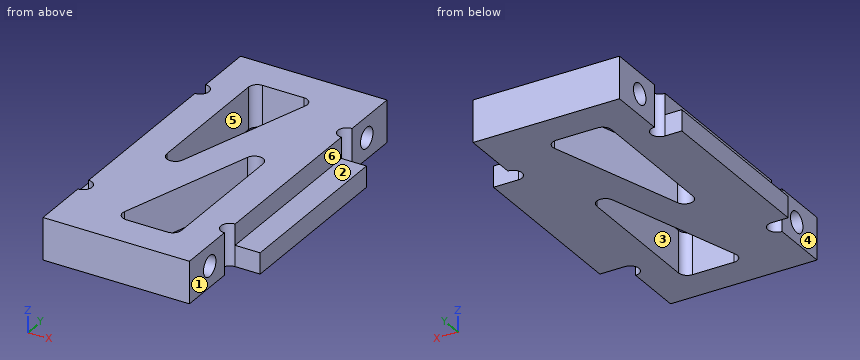
Autodesk Inventor part; units mm, degrees
ref_plane "YZ Plane" through (0, 0, 0) normal (1, 0, 0) x (0, 1, 0)
ref_plane "XZ Plane" through (0, 0, 0) normal (0, 1, 0) x (-1, 0, 0)
ref_plane "XY Plane" through (0, 0, 0) normal (0, 0, 1) x (1, 0, 0)
sketch "スケッチ1" plane through (0, 0, 0) normal (0, 0, 1) x (1, 0, 0)
  line L0 (-8.75, -19.5) -> (8.75, -19.5) construction
  line L1 (8.75, -19.5) -> (8.75, 19.5) construction
  line L2 (8.75, 19.5) -> (-8.75, 19.5) construction
  line L3 (-8.75, 19.5) -> (-8.75, -19.5) construction
  line L4 (-8.75, -19.5) -> (8.75, 19.5) construction
  line L5 (8.75, -19.5) -> (-8.75, 19.5) construction
  line L6 (-8.75, 10.5) -> (-8.75, 19.5) construction
  line L7 (-8.75, 19.5) -> (8.75, 19.5)
  line L8 (8.75, 19.5) -> (8.75, 10.5) construction
  line L9 (-8.75, 10.5) -> (-10.75, 10.5)
  line L10 (-10.75, 10.5) -> (-10.75, -10.5)
  line L11 (-10.75, -10.5) -> (-8.75, -10.5)
  line L12 (-8.75, -10.5) -> (-8.75, -19.5) construction
  line L13 (-8.75, -19.5) -> (8.75, -19.5)
  line L14 (8.75, -19.5) -> (8.75, -10.5) construction
  line L15 (8.75, -10.5) -> (11.75, -10.5)
  line L16 (11.75, -10.5) -> (11.75, 10.5)
  line L17 (11.75, 10.5) -> (8.75, 10.5)
  line L18 (0, 0) -> (11.75, 0) construction
  circle A0 centre (-8.75, 11.55) radius 1.05 construction
  circle A1 centre (-8.75, -11.55) radius 1.05 construction
  circle A2 centre (8.75, 11.55) radius 1.05 construction
  circle A3 centre (8.75, -11.55) radius 1.05 construction
  line L19 (-8.75, 19.5) -> (-8.75, 12.6)
  arc A4 (-8.75, 10.5) -> (-8.75, 12.6) centre (-8.75, 11.55) ccw
  arc A5 (-8.75, -12.6) -> (-8.75, -10.5) centre (-8.75, -11.55) ccw
  line L20 (-8.75, -12.6) -> (-8.75, -19.5)
  line L21 (8.75, 12.6) -> (8.75, 19.5)
  arc A6 (8.75, 12.6) -> (8.75, 10.5) centre (8.75, 11.55) ccw
  line L22 (8.75, -12.6) -> (8.75, -19.5)
  arc A7 (8.75, -10.5) -> (8.75, -12.6) centre (8.75, -11.55) ccw
  dimension "d21" = 2
  dimension "d23" = 3
  dimension "d30" = 17.5
  dimension "d48" = 9
  dimension "d49" = 39
  dimension "d50" = 2.1
extrude "押し出し1" add sketch "スケッチ1" along normal blind 5
sketch "スケッチ2" plane through (8.75, -19.5, 0) normal (1, 0, 0) x (0, 0, -1)
  line L0 (0, 0) -> (-5, 0)
  line L1 (0, 39) -> (-5, 39)
  point P0 (0, 19.5)
  point P1 (-2.5, 4)
  point P2 (-2.5, 35)
  point P3 (-2.5, 0)
  dimension "d53" = 4
  dimension "d54" = 4
hole "穴1" at (8.75, -15.5, 2.5) at (8.75, 15.5, 2.5) direction (-1, 0, 0) diameter 2.459 depth 2.5 tip angle 118
mirror "ミラー1" about plane through (0, 0, 0) normal (1, 0, 0) of "穴1"
sketch "スケッチ3" plane through (0, 0, 5) normal (0, 0, 1) x (1, 0, 0)
  line L0 (8.75, 12.6) -> (8.75, 19.5)
  line L1 (-8.75, 19.5) -> (-8.75, 12.6)
  line L2 (-13.3307, 15.6684) -> (-8.75, 15.6684)
  line L3 (-8.75, 15.6684) -> (-8.75, -16.7148)
  line L4 (-8.75, -16.7148) -> (-13.3307, -16.7148)
  line L5 (-13.3307, -16.7148) -> (-13.3307, 15.6684)
  line L6 (14.2214, 11.55) -> (8.75, 11.55)
  line L7 (8.75, 11.55) -> (8.75, -15.9078)
  line L8 (8.75, -15.9078) -> (14.2214, -15.9078)
  line L9 (14.2214, -15.9078) -> (14.2214, 11.55)
  point P0 (0, 0)
extrude "押し出し2" cut sketch "スケッチ3" against normal blind 2.5
sketch "スケッチ4" plane through (0, 0, 5) normal (0, 0, 1) x (1, 0, 0)
  line L0 (8.75, 12.6) -> (8.75, 19.5)
  line L1 (8.75, 19.5) -> (-8.75, 19.5)
  line L2 (-8.75, -12.6) -> (-8.75, -19.5)
  line L3 (-8.75, -19.5) -> (8.75, -19.5)
  line L4 (-4.75, 15.5) -> (4.75, 15.5) construction
  line L5 (4.75, 15.5) -> (4.75, -15.5) construction
  line L6 (4.75, -15.5) -> (-4.75, -15.5) construction
  line L7 (-4.75, -15.5) -> (-4.75, 15.5) construction
  line L8 (4.75, 15.5) -> (-4.75, -15.5) construction
  line L9 (2.6582, 15.5) -> (-4.75, 15.5)
  line L10 (-4.75, 15.5) -> (-4.75, -8.6741)
  line L11 (-4.75, -8.6741) -> (2.6582, 15.5)
  line L12 (-2.6582, -15.5) -> (4.75, -15.5)
  line L13 (4.75, -15.5) -> (4.75, 8.6741)
  line L14 (4.75, 8.6741) -> (-2.6582, -15.5)
  point P0 (0, 0)
  dimension "d64" = 4
  dimension "d65" = 4
  dimension "d66" = 4
  dimension "d67" = 4
  dimension "d68" = 4
extrude "押し出し3" cut sketch "スケッチ4" against normal blind 5
fillet "フィレット1" radius 1.05 6 edges at (-2.6582, -15.5, 2.5) (-4.75, 15.5, 2.5) (2.6582, 15.5, 2.5) (4.75, 8.6741, 2.5) (-4.75, -8.6741, 2.5) (4.75, -15.5, 2.5)
equation "\"d48\" = d26 + d35"
equation "\"d49\" = d38"
equation "\"d66\" = d65"
equation "\"d68\" = d67"
properties part number "胴体_メインフレーム_1_12" material "アセタール樹脂、黒"
Input: part model. Units: mm. Frame: model coordinates. Face numbers are marked on the shaded views. A direction names the side the tool comes from. Round coordinates to 2 decimals unless told otherwise and drop trailing zeros. Loops run counter-clockwise (first coordinate to the right, second up) from the corner with the lowest first, then second, coordinate; pieces in that order, holes last. Notation, with made-up numbers: (-11, 7) -> (30, 7) arc R19 cw to (30, 32) -> close; hole circle Ø9 at (-20, -31). An arc over 180 degrees is marked (long way). Answer as a JSON object with one key per item and string values. Group by question number.
1) Section query A-A on z = 0.45. Output: boundary loops of the cut face in (x, y), plus the area to 3 significant figures.
2) Draft query along X for the marked faces 1, 2 and 3. Return one class per face: +X half, -X half, draft (parallel to the pull), parting line (faces both ways), or undercut.
3) Reachability of the marked faces 4, 5 and 6 from +Z, -Z, +X, -X, +Y, -Y: full face, straight path, thin tool, end or side. Return the list, or none.
4) Section query C-C on z = 4.5. Output: boundary loops of the cut face in (x, y), plus the area to 3 significant figures.
5) Section query D-D on x = 10.75. Output: boundary loops of the cut face in (y, z), plus the area to 3 significant figures.
6) Section query B-B on y = 11.55. Output: boundary loops of the cut face in (x, z).
7) Pin query (flat end, axial travel): pin 1 (0.6 mm diameter, centred on x = -10, z = 1, fed in from +Y); pin 2 (3 mm diameter, centred on y = -15.5, z = 2.5, fed in from +X); pin 3 (1 mm diameter, centred on x = -10, y = 4, fed in from +Z). Return the tip coordinate at first contact, or that it passes through.
8) Ray query, L1, parallel to Z at x = 8.1, y = 15.5; L2, parallel to Y at x = -6.9, z = 2.5; L3, parallel to Y at x = 8, z = 3.25. Return the intervals inside material, ascending.
Reply:
{
 "1": {"outline": "(-10.75, -10.5) -> (-8.75, -10.5) arc R1.05 cw to (-8.75, -12.6) -> (-8.75, -19.5) -> (8.75, -19.5) -> (8.75, -12.6) arc R1.05 cw to (8.75, -10.5) -> (11.75, -10.5) -> (11.75, 10.5) -> (8.75, 10.5) arc R1.05 cw to (8.75, 12.6) -> (8.75, 19.5) -> (-8.75, 19.5) -> (-8.75, 12.6) arc R1.05 cw to (-8.75, 10.5) -> (-10.75, 10.5) -> close; hole (-4.75, -1.66) arc R1.05 ccw to (-2.7, -1.97) -> (2.24, 14.14) arc R1.05 ccw to (1.24, 15.5) -> (-3.7, 15.5) arc R1.05 ccw to (-4.75, 14.45) -> close; hole (-2.24, -14.14) arc R1.05 ccw to (-1.24, -15.5) -> (3.7, -15.5) arc R1.05 ccw to (4.75, -14.45) -> (4.75, 1.66) arc R1.05 ccw to (2.7, 1.97) -> close", "area": "614 mm2"},
 "2": {"face 1": "+X half", "face 2": "draft", "face 3": "undercut"},
 "3": {"face 4": "+Z, -Z, -X, -Y", "face 5": "+Z, -Z", "face 6": "+Z, +X, +Y, -Y"},
 "4": {"outline": "(-8.75, -19.5) -> (8.75, -19.5) -> (8.75, -12.6) arc R1.05 cw to (8.75, -10.5) -> (8.75, 10.5) arc R1.05 cw to (8.75, 12.6) -> (8.75, 19.5) -> (-8.75, 19.5) -> (-8.75, 12.6) arc R1.05 cw to (-8.75, 10.5) -> (-8.75, -10.5) arc R1.05 cw to (-8.75, -12.6) -> close; hole (-4.75, -1.66) arc R1.05 ccw to (-2.7, -1.97) -> (2.24, 14.14) arc R1.05 ccw to (1.24, 15.5) -> (-3.7, 15.5) arc R1.05 ccw to (-4.75, 14.45) -> close; hole (-2.24, -14.14) arc R1.05 ccw to (-1.24, -15.5) -> (3.7, -15.5) arc R1.05 ccw to (4.75, -14.45) -> (4.75, 1.66) arc R1.05 ccw to (2.7, 1.97) -> close", "area": "509 mm2"},
 "5": {"outline": "(-10.5, 0) -> (10.5, 0) -> (10.5, 2.5) -> (-10.5, 2.5) -> close", "area": "52.5 mm2"},
 "6": {"outline": "(-7.7, 0) -> (-4.75, 0) -> (-4.75, 5) -> (-7.7, 5) -> close; (1.45, 0) -> (7.7, 0) -> (7.7, 5) -> (1.45, 5) -> close"},
 "7": {"pin 1": "stops at y = 10.5", "pin 2": "stops at x = 8.75", "pin 3": "stops at z = 2.5"},
 "8": {"L1": "z = 0 to 1.27, 3.73 to 5", "L2": "y = -19.5 to -16.73, -14.27 to 14.27, 16.73 to 19.5", "L3": "y = -19.5 to -16.47, -14.53 to -12.28, -10.82 to 10.82, 12.28 to 14.53, 16.47 to 19.5"}
}
